```python
from build123d import *

# Parameters (mm, degrees)
SKETCH1_R                = 3.175
SKETCH1_R_2              = 2.54
BOSS_EXTRUDE1_DEPTH      = 50.8
BOSS_EXTRUDE2_DEPTH      = 0.508
BOSS_EXTRUDE2_DEPTH_BACK = 2.54
SKETCH2_R                = 2.54
BOSS_EXTRUDE3_START      = -48.26
SKETCH3_R                = 0.537131422
BOSS_EXTRUDE3_DEPTH      = 60.96


with BuildPart() as part:
    # Sketch1 → Boss-Extrude1 (new body)
    with BuildSketch(Plane.XY):
        Circle(SKETCH1_R)
        Circle(SKETCH1_R_2, mode=Mode.SUBTRACT)
    extrude(amount=BOSS_EXTRUDE1_DEPTH)

    # Sketch2 → Boss-Extrude2 (add, two sides: drawn at the far end of the back side and taken through both)
    with BuildSketch(Plane.XY.offset(50.8).offset(-BOSS_EXTRUDE2_DEPTH_BACK)):
        Circle(SKETCH2_R)
    extrude(amount=BOSS_EXTRUDE2_DEPTH + BOSS_EXTRUDE2_DEPTH_BACK)

    # Sketch3 → Boss-Extrude3 (add)
    with BuildSketch(Plane(origin=(0, 0, 0), x_dir=(-1, 0, 0), z_dir=(0, 0, -1)).offset(BOSS_EXTRUDE3_START)):
        with Locations(Location((0, 0, 0), (0, 0, 180))):
            Circle(SKETCH3_R)
    extrude(amount=BOSS_EXTRUDE3_DEPTH)


solid = part.part
```
The model under review builds one solid part; all positions refer to its coordinate system, in mm. A direction names the side the tool comes from. Round coordinates to 2 decimals unless told otherwise and drop trailing zeros. Write each loop counter-clockwise with the first axis right and the second up, starting at its lowest first coordinate (ties: lowest second). Pieces come first, ordered by that corner, then holes. Notation, with made-up numbers: (2.5, 49.25) - (60.5, 49.25) arc R7 ccw to (60.5, 60.25) - close; hole circle Ø2 at (37, 81.25). An arc over 180 degrees is marked (long way). Use one line per item in the form item = value.
Q1. Insertion check: pin 1 Ø1.5 at (y, z) = (1.5, 37.5) entering from +X; pin 2 Ø2 at (y, z) = (-1.5, 26) entering from -X; pin 3 Ø1.5 at (x, y) = (-1.5, 2) entering from -Z. Each pin has a flat end and moves straight along its axis. Give the tip position at first contact, or say it passes through.
Answer key:
pin_1 = 3.09
pin_2 = -3.14
pin_3 = 0
Q2. Consider section B-B (y = 0). State the section outline as (x, z) points (3 decimals), and give its area (3 significant figures).
Answer key:
outline = (-3.175, 0) - (-2.54, 0) - (-2.54, 48.26) - (-0.537, 48.26) - (-0.537, -12.7) - (0.537, -12.7) - (0.537, 48.26) - (2.54, 48.26) - (2.54, 0) - (3.175, 0) - (3.175, 50.8) - (2.54, 50.8) - (2.54, 51.308) - (-2.54, 51.308) - (-2.54, 50.8) - (-3.175, 50.8) - close
area = 145 mm2
Q3. Consider section A-A (z = 27). State the section outline as (x, y) points (3 decimals), and give its area (3 significant figures).
Answer key:
outline = circle Ø6.35 at (0, 0); circle Ø1.074 at (0, 0); hole circle Ø5.08 at (0, 0)
area = 12.3 mm2
Q4. Draft analysis for pull direction X (two halves, no side actions). For faces 4 (the cylindrical face through (-0.537, -0.024, 18.207)), 5 (the cylindrical face through (-0.69, -3.1, 25.04)), 6 (the flat face through (0, 0, -12.7)), state which applies: +X half, -X half, draft (parallel to the pull), parting line (faces both ways), or undercut.
Answer key:
face_4 = undercut
face_5 = parting line
face_6 = draft
Q5. For line 1 (Y direction, x = 0, z = 32.5) (3 decimals); line 2 (Z direction, x = 0.25, y = -2); line 3 (X direction, y = -1, z = 9.5), list the stretches that pass through material, from the lowest coordinate up. Write a range as [from, to].
Answer key:
line_1 = [-3.175, -2.54], [-0.537, 0.537], [2.54, 3.175]
line_2 = [48.26, 51.31]
line_3 = [-3.01, -2.33], [2.33, 3.01]
Q6. Tool access review of faces 1 (the flat face through (0, 3, 50.8)), 2 (the flat face through (0, 0, 51.308)), 3 (the flat face through (0, 1, 48.26)): name each direction out of +Z, -Z, +X, -X, +Y, -Y from which nothing blocks a thin tool from reaching the whole face with its end or side.
Answer key:
face_1 = +Z
face_2 = +Z, +X, -X, +Y, -Y
face_3 = -Z
